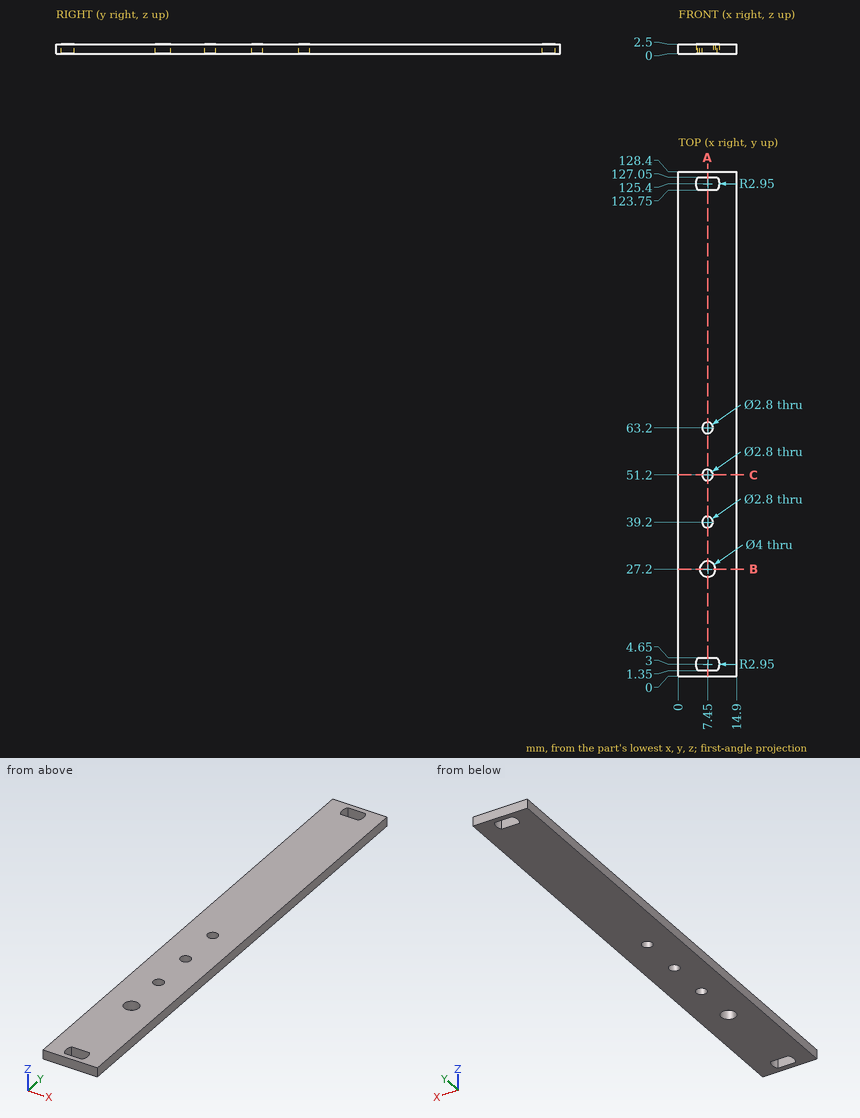
Design review of the part shown in the three views and the two pictorial views. Dimensions are in mm from the part's minimum x, y and z. Coordinates: 2 decimals unless noted, no trailing zeros. Loops run counter-clockwise (first coordinate to the right, second up) from the corner with the lowest first, then second, coordinate; pieces in that order, holes last.
(1) Consider section A-A, the plane x = 7.45. Give the boundary of the cut face in (y, z), plus the area to 4 significant figures.
Determined:
outline: (0, 0) - (1.35, 0) - (1.35, 2.5) - (0, 2.5) - close; (4.65, 0) - (25.2, 0) - (25.2, 2.5) - (4.65, 2.5) - close; (29.2, 0) - (37.8, 0) - (37.8, 2.5) - (29.2, 2.5) - close; (40.6, 0) - (49.8, 0) - (49.8, 2.5) - (40.6, 2.5) - close; (52.6, 0) - (61.8, 0) - (61.8, 2.5) - (52.6, 2.5) - close; (64.6, 0) - (123.75, 0) - (123.75, 2.5) - (64.6, 2.5) - close; (127.05, 0) - (128.4, 0) - (128.4, 2.5) - (127.05, 2.5) - close
area: 273.5 mm2
(2) Consider section C-C, the plane y = 51.2. Give the boundary of the cut face in (x, z).
Determined:
outline: (0, 0) - (6.05, 0) - (6.05, 2.5) - (0, 2.5) - close; (8.85, 0) - (14.9, 0) - (14.9, 2.5) - (8.85, 2.5) - close
(3) Wall thickness on L1, parallel to Y at x = 9.5, z = 1.05: over which ranges is the line inside the solid? List them lowest first.
Determined:
L1: y = 0 to 1.35, 4.65 to 123.75, 127.05 to 128.4
(4) Consider section B-B, the plane y = 27.2. Give the boundary of the cut face in (x, z), plus the area to 4 significant figures.
Determined:
outline: (0, 0) - (5.45, 0) - (5.45, 2.5) - (0, 2.5) - close; (9.45, 0) - (14.9, 0) - (14.9, 2.5) - (9.45, 2.5) - close
area: 27.25 mm2
